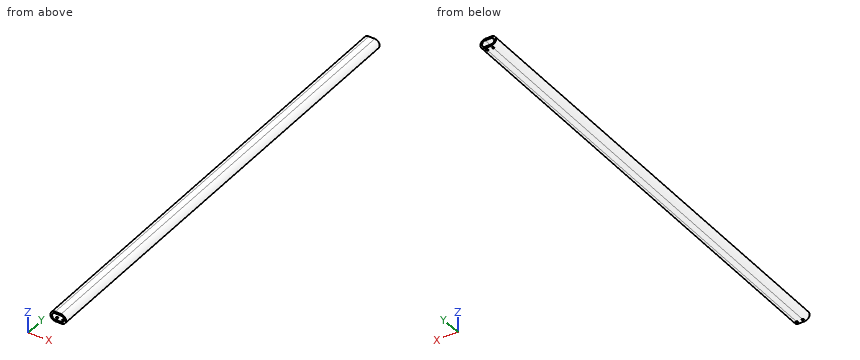
```python
from build123d import *

# Parameters (mm, degrees)
BOSS_EXTRUDE1_DEPTH = 2997.2
SKETCH2_R           = 6.35
CUT_EXTRUDE1_DEPTH  = 25.4


with BuildPart() as part:
    # Sketch1 → Boss-Extrude1 (new body)
    with BuildSketch(Plane(origin=(0, 0, 0), x_dir=(1, 0, 0), z_dir=(0, 1, 0))):
        with BuildLine():
            Line((0, 31.75), (38.1, 31.75))
            ThreePointArc((38.1, 31.75), (69.85, 0), (38.1, -31.75))
            Line((38.1, -31.75), (0, -31.75))
            ThreePointArc((0, -31.75), (-31.75, 0), (0, 31.75))
        make_face()
        with BuildLine():
            Line((0, 20.304779167), (38.1, 20.304779167))
            ThreePointArc((38.1, 20.304779167), (58.404779167, 0), (38.1, -20.304779167))
            Line((38.1, -20.304779167), (0, -20.304779167))
            ThreePointArc((0, -20.304779167), (-20.304779167, 0), (0, 20.304779167))
        make_face(mode=Mode.SUBTRACT)
    extrude(amount=BOSS_EXTRUDE1_DEPTH)

    # Sketch2 → Cut-Extrude1 (cut)
    with BuildSketch(Plane(origin=(0, 0, -31.75), x_dir=(-1, 0, 0), z_dir=(0, 0, -1))):
        with Locations((-38.1, 19.05)):
            Circle(SKETCH2_R)
        with Locations((0, 19.05)):
            Circle(SKETCH2_R)
        with Locations((-38.1, 2978.15)):
            Circle(SKETCH2_R)
        with Locations((0, 2978.15)):
            Circle(SKETCH2_R)
    extrude(amount=-CUT_EXTRUDE1_DEPTH, mode=Mode.SUBTRACT)


solid = part.part
```
Model file for the job. Use its own axes, mm. Give positions to 0.01 mm unless a question says otherwise; leave off trailing zeros. Loops run counter-clockwise (first coordinate to the right, second up) from the corner with the lowest first, then second, coordinate; pieces in that order, holes last. Notation, with made-up numbers: M 51,80.25 L 61,80.25 A23 cw 61,110.25 Z; hole C -31,72 d3. An arc over 180 degrees is marked long. Use one line per item in the form item = value.
Item 1: Slice it at B-B on z = -4.5. List the corners of the cut face in (x, y), and give its area (3 significant figures).
Filled in:
outline = M -31.43,0 L -19.8,0 L -19.8,2997.2 L -31.43,2997.2 Z; M 57.9,0 L 69.53,0 L 69.53,2997.2 L 57.9,2997.2 Z
area = 69,700 mm^2
Item 2: Flat gauge pins, fed straight in: pin 1 Ø1.5 at (y, z) = (569, -2) entering from -X; pin 2 Ø7.5 at (x, y) = (38.1, 2978.15) entering from -Z; pin 3 Ø10 at (y, z) = (734.5, 1.5) entering from +X. Where does each tip first touch, or does it go through?
Filled in:
pin_1 = -31.73
pin_2 = 19.96
pin_3 = 69.85
Item 3: Drill centre lines: L1, parallel to X at y = 2978.15, z = -24.5; L2, parallel to Y at x = 38.1, z = -25.75; L3, parallel to Z at x = 12, y = 2639. Where is each one in solid material? Low to high.
Filled in:
L1 = -20.19 to -6.35, 6.35 to 31.75, 44.45 to 58.29
L2 = 0 to 12.7, 25.4 to 2971.8, 2984.5 to 2997.2
L3 = -31.75 to -20.3, 20.3 to 31.75
Item 4: Slice it at A-A on y = 211. List the corners of the cut face in (x, z), and give its area (3 significant figures).
Filled in:
outline = M 0,-31.75 L 38.1,-31.75 A31.75 ccw 38.1,31.75 L 0,31.75 A31.75 ccw Z; hole M 0,-20.3 L 38.1,-20.3 A20.3 ccw 38.1,20.3 L 0,20.3 A20.3 ccw Z
area = 2,740 mm^2
